```python
from build123d import *

# Parameters (mm, degrees)
SKETCH1_R           = 35.56
BOSS_EXTRUDE1_DEPTH = 6.35
SKETCH3_R           = 1.905
CUT_EXTRUDE1_DEPTH  = 6.35
SKETCH4_R           = 5.08
SKETCH4_R_2         = 2.54
BOSS_EXTRUDE2_DEPTH = 8.89
SKETCH5_R           = 1.5
CUT_EXTRUDE2_DEPTH  = 10
SKETCH6_R           = 3.175
CUT_EXTRUDE3_DEPTH  = 8.89
CUT_EXTRUDE4_START  = 40.64
SKETCH8_R           = 1.7526
CUT_EXTRUDE4_DEPTH  = 17.78
CIRPATTERN1_COUNT   = 4


with BuildPart() as part:
    # Sketch1 → Boss-Extrude1 (new body)
    with BuildSketch(Plane(origin=(0, 0, 0), x_dir=(1, 0, 0), z_dir=(0, 1, 0))):
        with Locations(Location((0, 0, 0), (0, 0, 270))):
            Circle(SKETCH1_R)
    extrude(amount=BOSS_EXTRUDE1_DEPTH)

    # Sketch3 → Cut-Extrude1 (cut)
    with BuildSketch(Plane(origin=(0, 6.35, 0), x_dir=(1, 0, 0), z_dir=(0, 1, 0))):
        with Locations(Location((-12.7, 0, 0), (0, 0, 270))):
            Circle(SKETCH3_R)
        with Locations(Location((12.7, 0, 0), (0, 0, 270))):
            Circle(SKETCH3_R)
    extrude(amount=-CUT_EXTRUDE1_DEPTH, mode=Mode.SUBTRACT)

    # Sketch4 → Boss-Extrude2 (add)
    with BuildSketch(Plane(origin=(0, 6.35, 0), x_dir=(1, 0, 0), z_dir=(0, 1, 0))):
        with Locations(Location((0, 18.7325, 0), (0, 0, 270))):
            Circle(SKETCH4_R)
        with Locations(Location((0, 18.7325, 0), (0, 0, 270))):
            Circle(SKETCH4_R_2, mode=Mode.SUBTRACT)
    boss_extrude2 = extrude(amount=BOSS_EXTRUDE2_DEPTH)

    # Mirror1: Boss-Extrude2 across plane
    add(boss_extrude2.mirror(Plane.XY))

    # Sketch5 → Cut-Extrude2 (cut)
    with BuildSketch(Plane(origin=(0, 6.35, 0), x_dir=(1, 0, 0), z_dir=(0, 1, 0))):
        with Locations(Location((0, 18.7325, 0), (0, 0, 270))):
            Circle(SKETCH5_R)
        with Locations(Location((0, -18.7325, 0), (0, 0, 270))):
            Circle(SKETCH5_R)
    extrude(amount=-CUT_EXTRUDE2_DEPTH, mode=Mode.SUBTRACT)

    # Sketch6 → Cut-Extrude3 (cut)
    with BuildSketch(Plane(origin=(0, 15.24, 0), x_dir=(1, 0, 0), z_dir=(0, 1, 0))):
        with Locations(Location((0, 18.7325, 0), (0, 0, 270))):
            Circle(SKETCH6_R)
        with Locations(Location((0, -18.7325, 0), (0, 0, 270))):
            Circle(SKETCH6_R)
    extrude(amount=-CUT_EXTRUDE3_DEPTH, mode=Mode.SUBTRACT)

    # Sketch8 → Cut-Extrude4 (cut)
    with BuildSketch(Plane(origin=(0, 0, 0), x_dir=(0, 0, -1), z_dir=(1, 0, 0)).offset(CUT_EXTRUDE4_START)):
        with Locations((0, 3.175)):
            Circle(SKETCH8_R)
    cut_extrude4 = extrude(amount=-CUT_EXTRUDE4_DEPTH, mode=Mode.SUBTRACT)

    # CirPattern1: Cut-Extrude4 ×4 about axis
    cirpattern1_axis = Axis((0, 0, 0), (0, 1, 0))
    for i in range(1, CIRPATTERN1_COUNT):
        add(cut_extrude4.rotate(cirpattern1_axis, i * 360 / CIRPATTERN1_COUNT), mode=Mode.SUBTRACT)


solid = part.part
```
Source: CAD feature listing. Evaluate the final solid. Frame: model axes, mm. A direction names the side the tool comes from. Round coordinates to 2 decimals unless told otherwise and drop trailing zeros. Loops run counter-clockwise (first coordinate to the right, second up) from the corner with the lowest first, then second, coordinate; pieces in that order, holes last. Notation, with made-up numbers: (15, 34.25) - (47, 34.25) arc R26 cw to (47, 63.25) - close; hole circle Ø7 at (-10.5, 61.25). An arc over 180 degrees is marked (long way). Use CSV: the item, a comma, the result in double quotes.
Q1. Ray query, line 1 along X through (y, z) = (4, 0) (3 decimals); line 2 along Y through (x, z) = (0, 29); line 3 along Y through (x, z) = (25, -2.5). Return the intervals inside material, ascending.
Reported:
line 1,"-22.86 to -14.605, -10.795 to 10.795, 14.605 to 22.86"
line 2,"0 to 1.42, 4.93 to 6.35"
line 3,"0 to 6.35"
Q2. Pin query (flat end, axial travel): pin 1 Ø3 at (x, y) = (0, 3.175) entering from -Z; pin 2 Ø3 at (x, y) = (0, 3.175) entering from +Z; pin 3 Ø8 at (y, z) = (4.5, 14) entering from +X (3 decimals). Return the tip coordinate at first contact, or that it passes through.
Reported:
pin 1,"z = -22.86"
pin 2,"z = 22.86"
pin 3,"x = 34.125"
Q3. Section query A-A, the plane x = -12.7. Output: boundary loops of the cut face in (y, z) (3 decimals).
Reported:
outline,"(0, -33.215) - (6.35, -33.215) - (6.35, -1.905) - (0, -1.905) - close; (0, 1.905) - (6.35, 1.905) - (6.35, 33.215) - (0, 33.215) - close"
Q4. Mould query, pull axis Y, two halves, no side actions, for faces 5 (the flat face through (0, 6.35, 0)), 6 (the flat face through (0, 3, 22.86)), 7 (the cylindrical face through (0.95, 10.86, 21.76)). Classes: pulls with the +Y half, pulls with the -Y half, needs draft (parallel to the pull), parting line crosses it, or undercut.
Reported:
face 5,"pulls with the +Y half"
face 6,"undercut"
face 7,"needs draft"
Q5. Reachability of faces 1 (the cylindrical face through (10.68, 3.13, 33.92)), 2 (the flat face through (22.86, 3, 0)), 3 (the flat face through (0, 3, -22.86)), 4 (the cylindrical face through (0.223, 10.733, -23.808)) from +Z, -Z, +X, -X, +Y, -Y: full face, straight path, thin tool, end or side. Return the list, or none.
Reported:
face 1,"+Y, -Y"
face 2,"+X"
face 3,"-Z"
face 4,"+Y"
Q6. Section query B-B, the plane z = 0. Output: boundary loops of the cut face in (x, y) (3 decimals).
Reported:
outline,"(-35.56, 0) - (-14.605, 0) - (-14.605, 6.35) - (-35.56, 6.35) - (-35.56, 4.928) - (-22.86, 4.928) - (-22.86, 1.422) - (-35.56, 1.422) - close; (-10.795, 0) - (10.795, 0) - (10.795, 6.35) - (-10.795, 6.35) - close; (14.605, 0) - (35.56, 0) - (35.56, 1.422) - (22.86, 1.422) - (22.86, 4.928) - (35.56, 4.928) - (35.56, 6.35) - (14.605, 6.35) - close"
Q7. Section query D-D, the plane z = -25.5. Output: boundary loops of the cut face in (x, y) (3 decimals), then the cut area to 3 significant figures.
Reported:
outline,"(-24.784, 0) - (24.784, 0) - (24.784, 6.35) - (-24.784, 6.35) - close; hole circle Ø3.505 at (0, 3.175)"
area,"305 mm^2"
Q8. Section query C-C, the plane y = 9.5. Give the number of separate pieces and of enclosed holes in the cut face, then the cut area to 3 significant figures.
Reported:
separate pieces,"2"
enclosed holes,"2"
area,"98.8 mm^2"
